```python
from build123d import *

# Parameters (mm, degrees)
PAD007_DEPTH     = 0.5
PAD008_DEPTH     = 1
SKETCH013_W      = 8.15
SKETCH013_H      = 0.5
PAD009_DEPTH     = 0.8
CHAMFER002_SIZE  = 0.5
HOLE_D           = 1.6
HOLE_DEPTH       = 25
HOLE_CSINK_D     = 2.5
HOLE_CSINK_ANGLE = 90
POCKET003_DEPTH  = 1.1
SKETCH016_R      = 4
POCKET004_DEPTH  = 5
POCKET005_DEPTH  = 0.5
CHAMFER006_SIZE2 = 1.3
CHAMFER006_SIZE  = 1.8


with BuildPart() as part:
    # Sketch011 (on Face14 of Binder001) → Pad007 (new body)
    with BuildSketch(Plane(origin=(0, 0, 0), x_dir=(1, 0, 0), z_dir=(0, 0, -1))):
        Polygon((16, -31), (16, 0), (15, 1), (0, 1), (-1, 0), (-1, -31), (0, -32), (15, -32), align=None)
    extrude(amount=PAD007_DEPTH)

    # Sketch012 (on Face10 of Pad007) → Pad008 (join)
    with BuildSketch(Plane(origin=(0, 0, -0.5), x_dir=(1, 0, 0), z_dir=(0, 0, -1))):
        Polygon((-1.3, 1.8), (-1.8, 1.3), (-1.8, -32.3), (-1.3, -32.8), (16.3, -32.8), (16.8, -32.3), (16.8, 1.3), (16.3, 1.8), align=None)
    extrude(amount=PAD008_DEPTH)

    # Sketch013 (on Face7 of Pad008) → Pad009 (join)
    with BuildSketch(Plane.XZ.offset(1)):
        with Locations((7.5, -0.25)):
            Rectangle(SKETCH013_W, SKETCH013_H)
    extrude(amount=PAD009_DEPTH)

    # Chamfer002
    chamfer002_edges = [part.edges().sort_by_distance(p)[0] for p in [
        (-1.55, -1.55, -1.5),
        (-1.8, 15.5, -1.5),
        (-1.55, 32.55, -1.5),
        (7.5, 32.8, -1.5),
        (16.55, 32.55, -1.5),
        (16.8, 15.5, -1.5),
        (16.55, -1.55, -1.5),
        (7.5, -1.8, -1.5),
    ]]
    chamfer(chamfer002_edges, length=CHAMFER002_SIZE)

    # Hole
    with Locations(Plane(origin=(0, 0, -1.5), x_dir=(1, 0, 0), z_dir=(0, 0, -1))):
        with Locations((2, -7), (13, -7), (2, -29), (13, -29)):
            CounterSinkHole(HOLE_D / 2, HOLE_CSINK_D / 2, depth=HOLE_DEPTH, counter_sink_angle=HOLE_CSINK_ANGLE)

    # Sketch015 (on Face9 of Hole) → Pocket003 (cut)
    with BuildSketch(Plane.XY):
        with BuildLine():
            Line((8.1, 16.58), (8.1, 18.32))
            ThreePointArc((8.1, 18.32), (8.041421, 18.461421), (7.9, 18.52))
            Line((7.9, 18.52), (6.9, 18.52))
            ThreePointArc((6.9, 18.52), (6.758579, 18.461421), (6.7, 18.32))
            Line((6.7, 18.32), (6.7, 16.58))
            ThreePointArc((6.7, 16.58), (6.758579, 16.438579), (6.9, 16.38))
            Line((6.9, 16.38), (7.9, 16.38))
            ThreePointArc((7.9, 16.38), (8.041421, 16.438579), (8.1, 16.58))
        make_face()
    extrude(amount=-POCKET003_DEPTH, mode=Mode.SUBTRACT)

    # Sketch016 (on Face11 of Pocket003) → Pocket004 (cut)
    with BuildSketch(Plane(origin=(0, 0, -1.5), x_dir=(1, 0, 0), z_dir=(0, 0, -1))):
        with Locations((7.5, -24)):
            Circle(SKETCH016_R)
    extrude(amount=-POCKET004_DEPTH, mode=Mode.SUBTRACT)

    # Sketch017 → Pocket005 (cut)
    with BuildSketch(Plane.XY):
        with BuildLine():
            ThreePointArc((3.045, 3.435), (2.275, 4.205), (1.505, 3.435))
            Line((1.505, 3.435), (1.505, 2.445))
            ThreePointArc((1.505, 2.445), (2.275, 1.675), (3.045, 2.445))
            Line((3.045, 3.435), (3.045, 2.445))
        make_face()
        with BuildLine():
            ThreePointArc((13.495, 3.435), (12.725, 4.205), (11.955, 3.435))
            Line((11.955, 3.435), (11.955, 2.445))
            ThreePointArc((11.955, 2.445), (12.725, 1.675), (13.495, 2.445))
            Line((13.495, 3.435), (13.495, 2.445))
        make_face()
    extrude(amount=-POCKET005_DEPTH, mode=Mode.SUBTRACT)

    # Chamfer006
    chamfer006_edges = [part.edges().sort_by_distance(p)[0] for p in [
        (3.5, 24, -1.5),
    ]]
    chamfer006_side = part.faces().sort_by_distance((7.5, 14.586368, -1.5))[0]
    chamfer(chamfer006_edges, length=CHAMFER006_SIZE, length2=CHAMFER006_SIZE2, reference=chamfer006_side)


solid = part.part
```
Here's how the part is built. I have some questions about the finished solid (model axes, mm). A direction names the side the tool comes from. Coordinates: 2 decimals unless noted, no trailing zeros. Write each loop counter-clockwise with the first axis right and the second up, starting at its lowest first coordinate (ties: lowest second). Pieces come first, ordered by that corner, then holes. Notation, with made-up numbers: (-10.5, 60) - (13.5, 60) arc R22 cw to (13.5, 88) - close; hole circle Ø2 at (74.25, 40). An arc over 180 degrees is marked (long way). One line per item, written item: value.
1) We'd pull the mould along X, two halves only. Please class faces 4 (the flat face through (13, 3, -0.5)), 5 (the flat face through (7, 15, -1.5)), 6 (the flat face through (-0.5, -0.5, -0.2)), 7 (the flat face through (15.5, -0.5, -0.2)): pulls with the +X half, pulls with the -X half, needs draft (parallel to the pull), parting line crosses it, or undercut.
Model answer:
face 4: undercut
face 5: needs draft
face 6: pulls with the -X half
face 7: pulls with the +X half
2) I'm going to push a flat-ended pin straight in: P1, Ø0.5, axis at x = 12.5, y = 2.5, coming from the +Z side. Where does the tip first touch, or does it pass through?
Model answer:
P1: stops at z = -0.5
3) Suppose I cut it at C-C on y = 7. Write out the boundary of the cut face in (x, z), and give its area (3 significant figures).
Model answer:
outline: (-1.8, -1) - (-1.3, -1.5) - (0.75, -1.5) - (1.2, -1.05) - (1.2, 0) - (-1, 0) - (-1, -0.5) - (-1.8, -0.5) - close; (2.8, -1.05) - (3.25, -1.5) - (11.75, -1.5) - (12.2, -1.05) - (12.2, 0) - (2.8, 0) - close; (13.8, -1.05) - (14.25, -1.5) - (16.3, -1.5) - (16.8, -1) - (16.8, -0.5) - (16, -0.5) - (16, 0) - (13.8, 0) - close
area: 21.6 mm²
4) On a 3-axis mill with a long thin cutter (end or side, diameter ignored), from which of +Z, -Z, +X, -X, +Y, -Y can I reach the whole of each face in a straight line? I mean faces 1 (the flat face through (7, 17, -1.1)), 2 (the flat face through (15.5, 31.5, -0.2)), 3 (the cylindrical face through (2.104, 28.207, -0.518)). Say none if no direction works.
Model answer:
face 1: +Z
face 2: +Z, +X, +Y
face 3: +Z, -Z
5) Suppose I cut it at D-D on y = 11. Write out the boundary of the cut face in (x, z), and give its area (4 significant figures).
Model answer:
outline: (-1.8, -1) - (-1.3, -1.5) - (16.3, -1.5) - (16.8, -1) - (16.8, -0.5) - (16, -0.5) - (16, 0) - (-1, 0) - (-1, -0.5) - (-1.8, -0.5) - close
area: 26.85 mm²
6) Suppose I cut it at A-A on y = 24. Write out the boundary of the cut face in (x, z), and give its area (3 significant figures).
Model answer:
outline: (-1.8, -1) - (-1.3, -1.5) - (1.7, -1.5) - (3.5, -0.2) - (3.5, 0) - (-1, 0) - (-1, -0.5) - (-1.8, -0.5) - close; (11.5, -0.2) - (13.3, -1.5) - (16.3, -1.5) - (16.8, -1) - (16.8, -0.5) - (16, -0.5) - (16, 0) - (11.5, 0) - close
area: 12.5 mm²
7) I need wall thicknesses on line 1 along Y through (x, z) = (7.5, -0.05); line 2 along X through (y, z) = (7, -0.4); line 3 along Y through (x, z) = (13, -0.7). Which ranges of each line are inside material? Lowest first, please.
Model answer:
line 1: y = -1.8 to 16.38, 18.52 to 20, 28 to 32
line 2: x = -1 to 1.2, 2.8 to 12.2, 13.8 to 16
line 3: y = -1.8 to 6.2, 7.8 to 28.2, 29.8 to 32.8
8) Suppose I cut it at B-B on x = 7.5. Write out the boundary of the cut face in (y, z).
Model answer:
outline: (-1.8, -1) - (-1.3, -1.5) - (18.2, -1.5) - (20, -0.2) - (20, 0) - (18.52, 0) - (18.52, -1.1) - (16.38, -1.1) - (16.38, 0) - (-1.8, 0) - close; (28, -0.2) - (29.8, -1.5) - (32.3, -1.5) - (32.8, -1) - (32.8, -0.5) - (32, -0.5) - (32, 0) - (28, 0) - close
